Design review of the part built by this model. Coordinates are the model's own, in mm. A direction names the side the tool comes from. Give positions to 0.01 mm unless a question says otherwise; leave off trailing zeros. Loops run counter-clockwise (first coordinate to the right, second up) from the corner with the lowest first, then second, coordinate; pieces in that order, holes last. Notation, with made-up numbers: M 55.25,77.5 L 85.25,77.5 A26 cw 85.25,106.5 Z; hole C 41,-11.5 d8. An arc over 180 degrees is marked long. Use CSV: the item, a comma, the result in double quotes.
from build123d import *

# Parameters (mm, degrees)
F1_DEPTH = 40
F3_DEPTH = 45.001


with BuildPart() as f1:
    # F0 (on Top) → F1 (new body)
    with BuildSketch(Plane.XY):
        Polygon((-45, 0), (0, 0), (0, 75), (-15, 75), (-15, 15), (-45, 15), align=None)
    extrude(amount=F1_DEPTH)

    # F2 (on face) → F3 (cut, through all)
    with BuildSketch(Plane.YZ):
        with BuildLine():
            Line((65, 26.000001), (25, 26.000001))
            ThreePointArc((25, 26.000001), (20, 21.000001), (25, 16.000001))
            Line((25, 16.000001), (65, 16.000001))
            ThreePointArc((65, 16.000001), (70, 21.000001), (65, 26.000001))
        make_face()
    extrude(amount=-F3_DEPTH, mode=Mode.SUBTRACT)


solid = f1.part
(1) We need section B-B on x = -3.5. State the section outline as (y, z) points.
A:
outline,"M 0,0 L 75,0 L 75,40 L 0,40 Z; hole M 25,16 L 65,16 A5 ccw 65,26 L 25,26 A5 ccw Z"
(2) We need section C-C on z = 20. State the section outline as (x, y) points, then the cut area to 3 significant figures.
A:
outline,"M -45,0 L 0,0 L 0,20.1 L -15,20.1 L -15,15 L -45,15 Z; M -15,69.9 L 0,69.9 L 0,75 L -15,75 Z"
area,"828 mm²"
(3) Machinability: for faces 1 (the flat face through (-13, 30, 40)), 2 (the flat face through (-15, 45, 15)), 3 (the cylindrical face through (-7, 20, 21)), which of the approach directions +Z, -Z, +X, -X, +Y, -Y give a long, thin tool a straight path to every point of the face, cutting with its end or side? Answer none if there is none.
A:
face 1,"+Z, +X, -X, +Y, -Y"
face 2,"+Z, -Z, -X, +Y"
face 3,"+X, -X"
(4) We need section A-A on y = 55. State the section outline as (x, z) points, then the cut area to 3 significant figures.
A:
outline,"M -15,0 L 0,0 L 0,16 L -15,16 Z; M -15,26 L 0,26 L 0,40 L -15,40 Z"
area,"450 mm²"
(5) Wall thickness on line 1 along Z through (x, y) = (-3, 54); line 2 along Y through (x, z) = (-41.5, 18); line 3 along Y through (x, z) = (-9.5, 22): over which ranges is each line inside the solid? List them lowest first. Write a range as [from, to].
A:
line 1,"[0, 16], [26, 40]"
line 2,"[0, 15]"
line 3,"[0, 20.1], [69.9, 75]"
(6) We need section D-D on z = 10.5. State the section outline as (x, y) points.
A:
outline,"M -45,0 L 0,0 L 0,75 L -15,75 L -15,15 L -45,15 Z"
(7) The part is to be moulded in two halves that separate along Y. For faces 4 (the flat face through (-23, 0, 20)), 5 (the flat face through (-7, 45, 16)), 6 (the flat face through (-30, 15, 20)), 7 (the cylindrical face through (-7, 70, 21)), say which applies: released by +Y, released by -Y, zero draft, split by the parting line, or undercut.
A:
face 4,"released by -Y"
face 5,"undercut"
face 6,"released by +Y"
face 7,"undercut"
(8) Clearance check with flat-ended pins moving along their axes: P1, Ø5, axis at x = -39.5, z = 35.5, coming from the +Y side; P2, Ø4, axis at y = 65, z = 8, coming from the -X side. State where each tip first meets the part, or that it passes through.
A:
P1,"y = 15"
P2,"x = -15"
